```python
from build123d import *

# Parameters (mm, degrees)
F1_DEPTH = 200
F2_W     = 8
F2_H     = 82.9011678715
F3_DEPTH = 19.5
F4_R     = 24.4008451418
F5_DEPTH = 15


with BuildPart() as f1:
    # F0 (on Front) → F1 (new body)
    with BuildSketch(Plane.XZ):
        with BuildLine():
            Line((0, 45.3068651259), (-12.3650406395, 45.3068651259))
            ThreePointArc((-12.3650406395, 45.3068651259), (-16.8699670467, 42.4761133979), (-16.2739621693, 37.1891203522))
            Line((-16.2739621693, 37.1891203522), (37.2513475231, -29.9190782446))
            Line((37.2513475231, -29.9190782446), (-17.7486524769, -29.9190782446))
            ThreePointArc((-17.7486524769, -29.9190782446), (-21.2841863828, -31.3835443387), (-22.7486524769, -34.9190782446))
            Line((-22.7486524769, -34.9190782446), (-22.7486524769, -38.4026915))
            ThreePointArc((-22.7486524769, -38.4026915), (-21.2841863828, -41.9382254059), (-17.7486524769, -43.4026915))
            Line((-17.7486524769, -43.4026915), (63.2359994792, -43.4026915))
            ThreePointArc((63.2359994792, -43.4026915), (67.7023811618, -40.6502311917), (67.2513475231, -35.4232653662))
            Line((67.2513475231, -35.4232653662), (29.0742767855, 16.0276582094))
            ThreePointArc((29.0742767855, 16.0276582094), (28.4873114519, 17.9667747875), (29.2668350391, 19.8368133922))
            Line((29.2668350391, 19.8368133922), (33.5585934884, 24.5428886656))
            ThreePointArc((33.5585934884, 24.5428886656), (34.3418720133, 26.5437627089), (33.5861795165, 28.5552176636))
            Line((33.5861795165, 28.5552176636), (19.6212582392, 44.2976946213))
            ThreePointArc((19.6212582392, 44.2976946213), (18.6073694579, 45.0429653147), (17.3770216384, 45.3068651259))
            Line((17.3770216384, 45.3068651259), (0, 45.3068651259))
        make_face()
    extrude(amount=F1_DEPTH)

    # F2 (on face) → F3 (cut)
    with BuildSketch(Plane.XY.offset(45.3068651259)):
        with Locations((-0.9822997963, -97.1923060715)):
            Rectangle(F2_W, F2_H)
    extrude(amount=-F3_DEPTH, mode=Mode.SUBTRACT)

    # F4 (on face) → F5 (cut)
    with BuildSketch(Plane(origin=(26.4204382833, 0, 19.6042144857), x_dir=(0, 1, 0), z_dir=(0.8030696088, 0, 0.5958852268))):
        with Locations((-103.3766940236, -30.9382844716)):
            Circle(F4_R)
    extrude(amount=-F5_DEPTH, mode=Mode.SUBTRACT)


solid = f1.part
```
The model under review builds one solid part; all positions refer to its coordinate system, in mm. A direction names the side the tool comes from. Round coordinates to 2 decimals unless told otherwise and drop trailing zeros. Loops run counter-clockwise (first coordinate to the right, second up) from the corner with the lowest first, then second, coordinate; pieces in that order, holes last. Notation, with made-up numbers: M 89,40.5 L 106,40.5 A16 cw 106,46.5 Z; hole C -5,76 d1. An arc over 180 degrees is marked long. Answer as a JSON object with one key per item and string values.
(1) Draft analysis for pull direction Z (two halves, no side actions). For faces 1 (the flat face through (10, -99, -29.919)), 2 (the flat face through (-1, -55.742, 36)), 3 (the cylindrical face through (67.667, -98.6, -40.719)), state which applies: released by +Z, released by -Z, zero draft, split by the parting line, or undercut.
Resolved:
{"face 1": "undercut", "face 2": "zero draft", "face 3": "split by the parting line"}
(2) Take a section at C-C on y = -91. Give the boundary of the cut face in (x, z), and give its area (3 significant figures).
Resolved:
{"outline": "M -22.75,-38.4 A5 ccw -17.75,-43.4 L 63.24,-43.4 A5 ccw 67.25,-35.42 L 57.39,-22.13 L 45.34,-31.07 L 20.28,2.71 L 32.33,11.65 L 29.07,16.03 A3 cw 29.27,19.84 L 33.56,24.54 A3 ccw 33.59,28.56 L 19.62,44.3 A3 ccw 17.38,45.31 L 3.02,45.31 L 3.02,25.81 L -4.98,25.81 L -4.98,45.31 L -12.37,45.31 A5 ccw -16.27,37.19 L 37.25,-29.92 L -17.75,-29.92 A5 ccw -22.75,-34.92 Z", "area": "2,790 mm²"}
(3) Take a section at B-B on x = 26. Count the separate pieces of the cut face and the enclosed holes in it, and give its area (3 significant figures).
Resolved:
{"separate pieces": "2", "enclosed holes": "1", "area": "12,800 mm²"}
(4) Clearance check with flat-ended pins moving along their axes: P1, Ø5, axis at y = -29.5, z = 16.5, coming from the +X side; P2, Ø21.5, axis at y = -94, z = 34.5, coming from the -X side; P3, Ø3, axis at y = -176.5, z = 22, coming from the -X side. State where each tip first meets the part, or that it passes through.
Resolved:
{"P1": "x = 30.58", "P2": "x = -17.37", "P3": "x = -5.36"}
(5) To check wall thickness, follow line 1 along Z through (x, y) = (32, -73); line 2 along Z through (x, y) = (-7.5, -99.5); line 3 along Z through (x, y) = (22.5, -50.5). State the ranges of each line that lie inside material, in increasing order.
Resolved:
{"line 1": "-43.4 to -29.92, -23.34 to 12.08, 22.83 to 30.34", "line 2": "-43.4 to -29.92, 26.19 to 45.31", "line 3": "-43.4 to -29.92, -11.42 to 41.05"}
(6) Take a section at A-A on y = -16.5. Give the boundary of the cut face in (x, z).
Resolved:
{"outline": "M -22.75,-38.4 A5 ccw -17.75,-43.4 L 63.24,-43.4 A5 ccw 67.25,-35.42 L 29.07,16.03 A3 cw 29.27,19.84 L 33.56,24.54 A3 ccw 33.59,28.56 L 19.62,44.3 A3 ccw 17.38,45.31 L -12.37,45.31 A5 ccw -16.27,37.19 L 37.25,-29.92 L -17.75,-29.92 A5 ccw -22.75,-34.92 Z"}
(7) Tool access review of faces 4 (the flat face through (10.114, -98.6, 4.105)), 5 (the flat face through (3.018, -98, 36)), 6 (the flat face through (32.61, -103.72, -13.91)), 7 (the flat face through (31.383, -98.6, 22.157)): name each direction out of +Z, -Z, +X, -X, +Y, -Y from which nothing blocks a thin tool from reaching the whole face with its end or side.
Resolved:
{"face 4": "-X, +Y, -Y", "face 5": "+Z", "face 6": "none", "face 7": "+X, +Y, -Y"}
